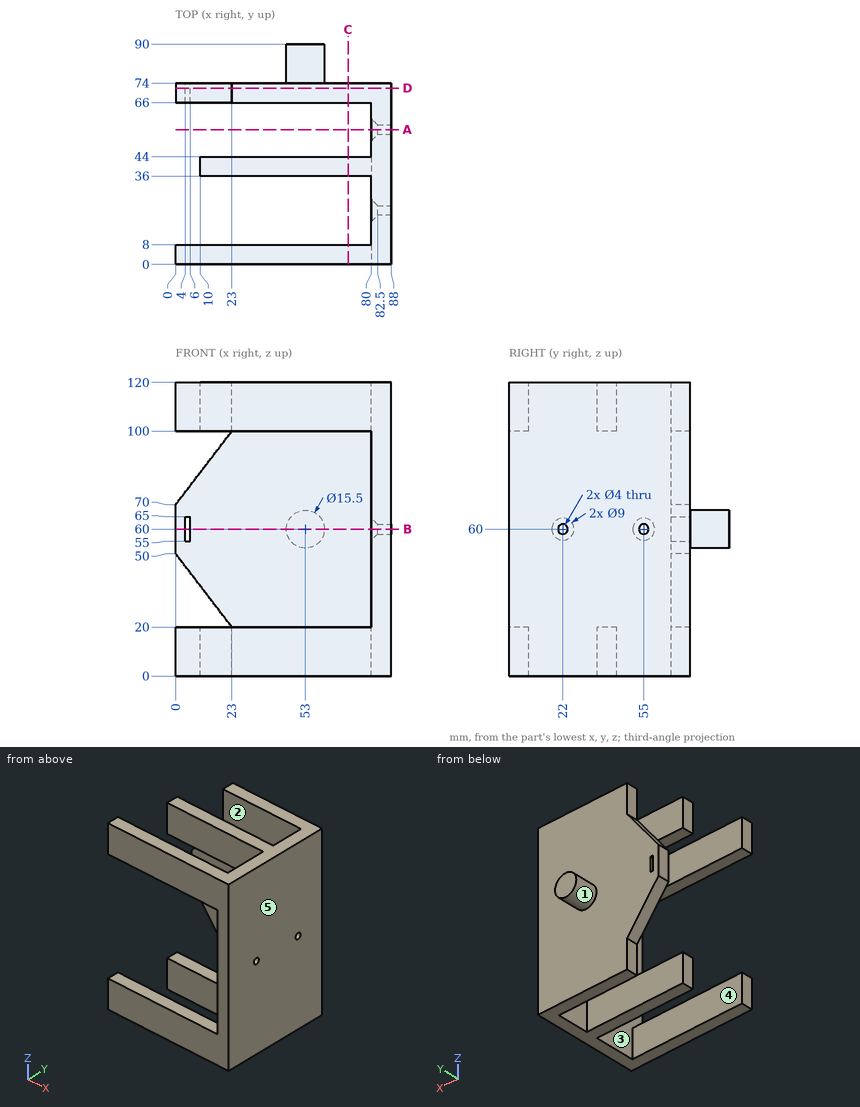
Design review of the part shown in the three views and the two pictorial views. Dimensions are in mm from the part's minimum x, y and z. A direction names the side the tool comes from. Round coordinates to 2 decimals unless told otherwise and drop trailing zeros. Write each loop counter-clockwise with the first axis right and the second up, starting at its lowest first coordinate (ties: lowest second). Pieces come first, ordered by that corner, then holes.
Item 1: For the marked faces 4 and 5, list the 3-axis set-ups (+Z, -Z, +X, -X, +Y, -Y) from which the entire face can be reached by the end or side of a thin tool; tool diameter is ignored.
Item 2: Consider section A-A on y = 55. Give the boundary of the cut face in (x, z).
Item 3: For pin 1 Ø20 at (y, z) = (49, 66.5) entering from -X; pin 2 Ø3 at (x, z) = (68.5, 46) entering from +Y; pin 3 Ø4 at (y, z) = (71.5, 8) entering from -X, all flat-tipped, find the tip position at first contact; note any pin that passes through.
Item 4: Wall thickness on L1, parallel to Y at x = 39, z = 12; L2, parallel to Y at x = 86, z = 60; L3, parallel to Z at x = 84, y = 22: over which ranges is each line inside the solid? List them lowest first.
Item 5: Draft analysis for pull direction Z (two halves, no side actions). For the marked faces 1, 2 and 3, state which applies: released by +Z, released by -Z, zero draft, split by the parting line, or undercut.
Item 6: Consider section B-B on z = 60. Give the boundary of the cut face in (x, y), and give its area (3 significant figures).
Item 7: Consider section C-C on x = 70.5. Give the boundary of the cut face in (y, z).
Item 8: Consider section D-D on y = 72. Give the boundary of the cut face in (x, z).
Check values:
1. face 4: +Z, -Z, -X
1. face 5: +Z, -Z, +X, +Y, -Y
2. outline: (80, 0) - (88, 0) - (88, 58) - (82.5, 58) - (80, 55.5) - close; (80, 64.5) - (82.5, 62) - (88, 62) - (88, 120) - (80, 120) - close
3. pin 1: stops at x = 80
3. pin 2: stops at y = 74
3. pin 3: stops at x = 23
4. L1: y = 0 to 8, 36 to 44, 66 to 74
4. L2: y = 0 to 20, 24 to 53, 57 to 74
4. L3: z = 0 to 58, 62 to 120
5. face 1: split by the parting line
5. face 2: zero draft
5. face 3: undercut
6. outline: (0, 66) - (4, 66) - (4, 74) - (0, 74) - close; (6, 66) - (80, 66) - (80, 59.5) - (82.5, 57) - (88, 57) - (88, 74) - (60.75, 74) - (60.75, 90) - (45.25, 90) - (45.25, 74) - (6, 74) - close; (80, 0) - (88, 0) - (88, 20) - (82.5, 20) - (80, 17.5) - close; (80, 26.5) - (82.5, 24) - (88, 24) - (88, 53) - (82.5, 53) - (80, 50.5) - close
6. area: 1,390 mm2
7. outline: (0, 0) - (8, 0) - (8, 20) - (0, 20) - close; (0, 100) - (8, 100) - (8, 120) - (0, 120) - close; (36, 0) - (44, 0) - (44, 20) - (36, 20) - close; (36, 100) - (44, 100) - (44, 120) - (36, 120) - close; (66, 0) - (74, 0) - (74, 120) - (66, 120) - close
8. outline: (0, 50) - (23, 20) - (23, 0) - (88, 0) - (88, 120) - (23, 120) - (23, 100) - (0, 70) - close; hole (4, 55) - (6, 55) - (6, 65) - (4, 65) - close
